from build123d import *

# Parameters (mm, degrees)
SKETCH2_R          = 30
ACRYLICBASE_DEPTH  = 1.5875
SKETCH3_W          = 5
SKETCH3_H          = 26
WHEELS_DEPTH       = 43.545042308
RELIEFS_R          = 2
SKETCH4_R          = 1.9304
CUT_EXTRUDE1_DEPTH = 43.545042308


with BuildPart() as part:
    # Sketch2 → AcrylicBase (new, symmetric)
    with BuildSketch(Plane(origin=(0, 0, 0), x_dir=(1, 0, 0), z_dir=(0, 1, 0))):
        with Locations(Location((0, 0, 0), (0, 0, 270))):
            Circle(SKETCH2_R)
    extrude(amount=ACRYLICBASE_DEPTH, both=True)

    # Sketch3 → wheels (cut, through all)
    with BuildSketch(Plane(origin=(0, 1.5875, 0), x_dir=(1, 0, 0), z_dir=(0, 1, 0))):
        with Locations((-20.657104633, 0)):
            Rectangle(SKETCH3_W, SKETCH3_H)
        with Locations((20.657104633, 0)):
            Rectangle(SKETCH3_W, SKETCH3_H)
    extrude(amount=-WHEELS_DEPTH, mode=Mode.SUBTRACT)

    # reliefs
    reliefs_edges = [part.edges().sort_by_distance(p)[0] for p in [
        (-23.157104633, 0, -13),
        (-18.157104633, 0, -13),
        (-18.157104633, 0, 13),
        (23.157104633, 0, -13),
        (23.157104633, 0, 13),
        (18.157104633, 0, 13),
        (18.157104633, 0, -13),
        (-23.157104633, 0, 13),
    ]]
    fillet(reliefs_edges, radius=RELIEFS_R)

    # Sketch4 → Cut-Extrude1 (cut, through all)
    with BuildSketch(Plane(origin=(0, 1.5875, 0), x_dir=(1, 0, 0), z_dir=(0, 1, 0))):
        with Locations(Location((-15, 20, 0), (0, 0, 270))):
            Circle(SKETCH4_R)
        with Locations(Location((-15, -20, 0), (0, 0, 270))):
            Circle(SKETCH4_R)
        with Locations(Location((15, -20, 0), (0, 0, 270))):
            Circle(SKETCH4_R)
        with Locations(Location((15, 20, 0), (0, 0, 270))):
            Circle(SKETCH4_R)
    extrude(amount=-CUT_EXTRUDE1_DEPTH, mode=Mode.SUBTRACT)


solid = part.part
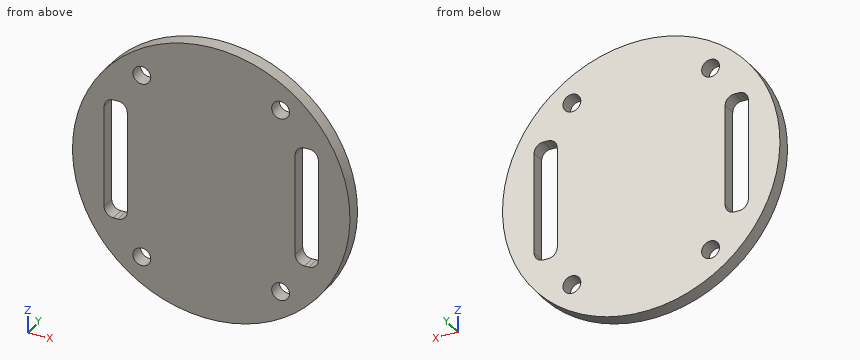
Read the model definition and answer for the solid it produces. Units are mm, in the model's axes. Coordinates: 2 decimals unless noted, no trailing zeros. Write each loop counter-clockwise with the first axis right and the second up, starting at its lowest first coordinate (ties: lowest second). Pieces come first, ordered by that corner, then holes. Notation, with made-up numbers: M 42,64.25 L 85,64.25 A33 cw 85,98.25 Z; hole C 41,47.25 d8. An arc over 180 degrees is marked long. Use a Markdown table: item, result.
Q1. Straight lines are drawn through the part: L1, parallel to X at y = 0.4, z = 20; L2, parallel to X at y = -0.45, z = -11; L3, parallel to Z at x = -20.5, y = -0.15. For each, find the intervals that lie inside material, in ascending order. Write a range as [from, to].
Answer block:
| item | result |
|---|---|
| L1 | x = [-22.36, -16.93], [-13.07, 13.07], [16.93, 22.36] |
| L2 | x = [-27.91, -23.16], [-18.16, 18.16], [23.16, 27.91] |
| L3 | z = [-21.9, -13], [13, 21.9] |
Q2. The part is cut by section B-B, the plane z = -20. Write down the section's boundary in (x, y), then the cut area to 3 significant figures.
Answer block:
| item | result |
|---|---|
| outline | M -22.36,-1.59 L -16.93,-1.59 L -16.93,1.59 L -22.36,1.59 Z; M -13.07,-1.59 L 13.07,-1.59 L 13.07,1.59 L -13.07,1.59 Z; M 16.93,-1.59 L 22.36,-1.59 L 22.36,1.59 L 16.93,1.59 Z |
| area | 117 mm2 |
Q3. The part is cut by section C-C, the plane x = 15. Write down the section's boundary in (y, z), then the cut area to 3 significant figures.
Answer block:
| item | result |
|---|---|
| outline | M -1.59,-25.98 L 1.59,-25.98 L 1.59,-21.93 L -1.59,-21.93 Z; M -1.59,-18.07 L 1.59,-18.07 L 1.59,18.07 L -1.59,18.07 Z; M -1.59,21.93 L 1.59,21.93 L 1.59,25.98 L -1.59,25.98 Z |
| area | 140 mm2 |
Q4. Each of these flat-tipped pins is pushed along its axis until it touches: pin 1 Ø1.6 at (y, z) = (-0.5, -3.5) entering from +X; pin 2 Ø0.8 at (x, y) = (-20.5, -0.5) entering from +Z; pin 3 Ø4.5 at (x, z) = (-15, -20) entering from -Y; pin 4 Ø1 at (x, y) = (-13.5, 0) entering from -Z. Where does it stop, or does it pass through?
Answer block:
| item | result |
|---|---|
| pin 1 | stops at x = 29.88 |
| pin 2 | stops at z = 22.27 |
| pin 3 | stops at y = -1.59 |
| pin 4 | stops at z = -27.04 |
Q5. The part is cut by section A-A, the plane y = 0.45. Write down the section's boundary in (x, z).
Answer block:
| item | result |
|---|---|
| outline | C 0,0 d60; hole M -23.16,-11 A2 ccw -21.16,-13 L -20.16,-13 A2 ccw -18.16,-11 L -18.16,11 A2 ccw -20.16,13 L -21.16,13 A2 ccw -23.16,11 Z; hole C -15,-20 d3.86; hole C -15,20 d3.86; hole C 15,-20 d3.86; hole C 15,20 d3.86; hole M 18.16,-11 A2 ccw 20.16,-13 L 21.16,-13 A2 ccw 23.16,-11 L 23.16,11 A2 ccw 21.16,13 L 20.16,13 A2 ccw 18.16,11 Z |
